Here's how the part is built. I have some questions about the finished solid (model axes, mm). Face numbers are marked on the shaded views. A direction names the side the tool comes from. Coordinates: 2 decimals unless noted, no trailing zeros. Write each loop counter-clockwise with the first axis right and the second up, starting at its lowest first coordinate (ties: lowest second). Pieces come first, ordered by that corner, then holes.
(1) Imagine slicing it at D-D, the plane y = -6. List the corners of the cut face in (x, z) for me, plus the area to 3 significant figures.
(2) Imagine slicing it at C-C, the plane y = -1. List the corners of the cut face in (x, z) for me.
(3) Which directions (+Z, -Z, +X, -X, +Y, -Y) give clear straight access to the entire face, cutting with the end or side of a thin tool? Please do the marked faces 1 and 2.
(4) For pin 1 Ø3 at (y, z) = (-5, -5) entering from +X; pin 2 Ø1 at (y, z) = (-6.5, 1) entering from +X; pin 3 Ø4 at (y, z) = (-3, 4.5) entering from -X, each with a flat end and sliding along its axis, tell me the tip position at first contact or that it passes through.
(5) Imagine slicing it at B-B, the plane z = 0. List the corners of the cut face in (x, y) for me.
(6) Please list where these lines run through material, in increasing order: probe 1 along Z at (x, y) = (0, -6); probe 2 along Z at (x, y) = (0, -1.8); probe 3 along Y at (x, z) = (0.5, 3.5).
(7) Thinking about a two-plate mould opening in Z: for the marked faces 3, 4, 5 and 6, which applies, released by +Z, released by -Z, zero draft, split by the parting line, or undercut?
(8) Imagine slicing it at A-A, the plane x = 0. List the corners of the cut face in (y, z) for me, plus the area to 3 significant figures.
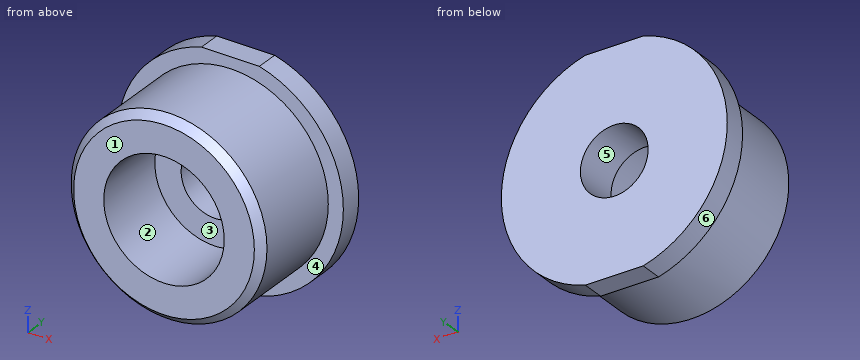
Autodesk Inventor part; units mm, degrees
ref_plane "YZ Plane" through (0, 0, 0) normal (1, 0, 0) x (0, 1, 0)
ref_plane "XZ Plane" through (0, 0, 0) normal (0, 1, 0) x (-1, 0, 0)
ref_plane "XY Plane" through (0, 0, 0) normal (0, 0, 1) x (1, 0, 0)
sketch "Sketch1" plane through (0, 0, 0) normal (0, 0, 1) x (1, 0, 0)
  line L0 (0, 0) -> (0, -9.8072)
  line L1 (2.25, 0) -> (7.5, 0)
  line L2 (7.5, 0) -> (7.5, -1.5)
  line L3 (7.5, -1.5) -> (6.5, -1.5)
  line L4 (6.5, -1.5) -> (6.5, -8)
  line L5 (6.5, -8) -> (4, -8)
  line L6 (4, -8) -> (4, -3)
  line L7 (2.25, -1) -> (2.25, -1)
  line L8 (2.25, -1) -> (2.25, 0)
  line L9 (2.25, -1) -> (2.25, -3)
  line L10 (2.25, -3) -> (4, -3)
  dimension "d1" = 4.5
  dimension "d2" = 8
  dimension "d3" = 13
  dimension "d4" = 1.5
  dimension "d6" = 15
  dimension "d19" = 2
  dimension "d20" = 4.5
  dimension "d21" = 8
  dimension "d22" = 2.5
  dimension "d25" = 5
  dimension "d26" = 1
revolve "Revolution1" add sketch "Sketch1" angle 360 about axis through (0, 0, 0) along (0, -1, 0)
sketch "Sketch2" plane through (0, 0, 0) normal (0, 1, 0) x (1, 0, 0)
  circle A0 centre (0, 0) radius 7.5
  line L0 (-1.9203, -7.25) -> (1.9203, -7.25)
  line L1 (1.9203, -7.25) -> (1.9203, 7.25)
  line L2 (1.9203, 7.25) -> (-1.9203, 7.25)
  line L3 (-1.9203, 7.25) -> (-1.9203, -7.25)
  point P0 (0, -7.25)
  point P1 (1.9203, -7.25)
  point P2 (-1.9203, 7.25)
  point P3 (1.9203, -7.25)
  point P4 (-1.9203, 7.25)
  dimension "d29" = 14.5
extrude "Extrusion1" cut sketch "Sketch2" against normal blind 10 contours L2 A0 | A0 L0
chamfer "Chamfer1" distance 0.5 angle 45 1 edges at (-6.5, -8, 0)
thread "Thread3"
equation "\"d1\" = d20"
properties part number "endcap"
Recorded:
1. outline: circle Ø13 at (0, 0); hole circle Ø8 at (0, 0)
1. area: 82.5 mm2
2. outline: (-1.92, -7.25) - (1.92, -7.25) arc R7.5 ccw to (1.92, 7.25) - (-1.92, 7.25) arc R7.5 ccw to start; hole circle Ø4.5 at (0, 0)
3. face 1: +Z, -Z, +X, -X, -Y
3. face 2: -Y
4. pin 1: stops at x = 5.48
4. pin 2: stops at x = 6.48
4. pin 3: stops at x = -6.79
5. outline: (-7.5, -1.5) - (-6.5, -1.5) - (-6.5, -7.5) - (-6, -8) - (-4, -8) - (-4, -3) - (-2.25, -3) - (-2.25, 0) - (-7.5, 0) - close; (2.25, -3) - (4, -3) - (4, -8) - (6, -8) - (6.5, -7.5) - (6.5, -1.5) - (7.5, -1.5) - (7.5, 0) - (2.25, 0) - close
6. probe 1: z = -6.5 to -4, 4 to 6.5
6. probe 2: z = -6.5 to -2.25, 2.25 to 6.5
6. probe 3: y = -3 to 0
7. face 3: undercut
7. face 4: zero draft
7. face 5: undercut
7. face 6: split by the parting line
8. outline: (-8, -6) - (-7.5, -6.5) - (-1.5, -6.5) - (-1.5, -7.25) - (0, -7.25) - (0, -2.25) - (-3, -2.25) - (-3, -4) - (-8, -4) - close; (-8, 4) - (-3, 4) - (-3, 2.25) - (0, 2.25) - (0, 7.25) - (-1.5, 7.25) - (-1.5, 6.5) - (-7.5, 6.5) - (-8, 6) - close
8. area: 52.5 mm2
